Check sheet for the modelled part. Datum: model origin and axes. Units: mm. A direction names the side the tool comes from. Round coordinates to 2 decimals unless told otherwise and drop trailing zeros. Order: outer loops, then holes, each group sorted by start corner. A loop starts at its lowest first (then second) coordinate and runs counter-clockwise, first axis right, second up. Notation, with made-up numbers: (76.25, 88.25) -> (87.25, 88.25) arc R31 ccw to (87.25, 119.25) -> close; hole circle Ø10 at (75, -30.5). An arc over 180 degrees is marked (long way). Answer in a Markdown table with one row per item.
```python
from build123d import *

# Parameters (mm, degrees)
SKETCH_1_W          = 60
SKETCH_1_H          = 20
SKETCH_1_W_2        = 58
SKETCH_1_H_2        = 18
EXTRUDE_1_DEPTH     = 320
SKETCH_2_R          = 2
CUT_EXTRUDE_1_DEPTH = 327.190128606
SKETCH_4_R          = 1.5
CUT_EXTRUDE_2_DEPTH = 327.190128606
SKETCH_5_R          = 10
SKETCH_5_R_2        = 12.5
CUT_EXTRUDE_3_DEPTH = 327.190128606


with BuildPart() as part:
    # 草图1 → 拉伸-薄壁1 (new body)
    with BuildSketch(Plane.XY):
        with Locations((30, 10)):
            Rectangle(SKETCH_1_W, SKETCH_1_H)
        with Locations((30, 10)):
            Rectangle(SKETCH_1_W_2, SKETCH_1_H_2, mode=Mode.SUBTRACT)
    extrude(amount=EXTRUDE_1_DEPTH)

    # 草图2 → 切除-拉伸1 (cut, through all)
    with BuildSketch(Plane(origin=(0, 20, 0), x_dir=(1, 0, 0), z_dir=(0, 1, 0))):
        with Locations(Location((5, -145, 0), (0, 0, 270))):
            Circle(SKETCH_2_R)
        with Locations(Location((5, -175, 0), (0, 0, 270))):
            Circle(SKETCH_2_R)
        with Locations(Location((55, -175, 0), (0, 0, 90))):
            Circle(SKETCH_2_R)
        with Locations(Location((55, -145, 0), (0, 0, 90))):
            Circle(SKETCH_2_R)
        with Locations(Location((5, -115, 0), (0, 0, 270))):
            Circle(SKETCH_2_R)
        with Locations(Location((5, -205, 0), (0, 0, 90))):
            Circle(SKETCH_2_R)
        with Locations(Location((55, -205, 0), (0, 0, 270))):
            Circle(SKETCH_2_R)
        with Locations(Location((55, -115, 0), (0, 0, 90))):
            Circle(SKETCH_2_R)
        with Locations(Location((5, -5, 0), (0, 0, 270))):
            Circle(SKETCH_2_R)
        with Locations(Location((55, -5, 0), (0, 0, 270))):
            Circle(SKETCH_2_R)
        with Locations(Location((55, -25, 0), (0, 0, 270))):
            Circle(SKETCH_2_R)
        with Locations(Location((5, -25, 0), (0, 0, 270))):
            Circle(SKETCH_2_R)
        with Locations(Location((5, -295, 0), (0, 0, 90))):
            Circle(SKETCH_2_R)
        with Locations(Location((55, -295, 0), (0, 0, 90))):
            Circle(SKETCH_2_R)
        with Locations(Location((55, -315, 0), (0, 0, 90))):
            Circle(SKETCH_2_R)
        with Locations(Location((5, -315, 0), (0, 0, 90))):
            Circle(SKETCH_2_R)
    extrude(amount=-CUT_EXTRUDE_1_DEPTH, mode=Mode.SUBTRACT)

    # 草图4 → 切除-拉伸2 (cut, through all)
    with BuildSketch(Plane(origin=(60, 0, 0), x_dir=(0, 0, -1), z_dir=(1, 0, 0))):
        with Locations((-315, 10)):
            Circle(SKETCH_4_R)
        with Locations((-295, 10)):
            Circle(SKETCH_4_R)
        with Locations(Location((-25, 10, 0), (0, 0, 180))):
            Circle(SKETCH_4_R)
        with Locations(Location((-5, 10, 0), (0, 0, 180))):
            Circle(SKETCH_4_R)
    extrude(amount=-CUT_EXTRUDE_2_DEPTH, mode=Mode.SUBTRACT)

    # 草图5 → 切除-拉伸3 (cut, through all)
    with BuildSketch(Plane(origin=(0, 20, 0), x_dir=(1, 0, 0), z_dir=(0, 1, 0))):
        with Locations(Location((30, -160, 0), (0, 0, 270))):
            Circle(SKETCH_5_R)
        with Locations(Location((30, -130, 0), (0, 0, 270))):
            Circle(SKETCH_5_R_2)
        with Locations(Location((30, -190, 0), (0, 0, 90))):
            Circle(SKETCH_5_R_2)
        with Locations(Location((30, -75, 0), (0, 0, 270))):
            Circle(SKETCH_5_R_2)
        with Locations(Location((30, -15, 0), (0, 0, 270))):
            Circle(SKETCH_5_R)
        with Locations(Location((30, -305, 0), (0, 0, 90))):
            Circle(SKETCH_5_R)
        with Locations(Location((30, -245, 0), (0, 0, 90))):
            Circle(SKETCH_5_R_2)
    extrude(amount=-CUT_EXTRUDE_3_DEPTH, mode=Mode.SUBTRACT)


solid = part.part
```
(1) Tool access check on faces 1 (the flat face through (16, 20, 158)), 2 (the flat face through (42, 1, 158)). Record the directions out of +Z, -Z, +X, -X, +Y, -Y that give a thin tool (end or side, any length) a straight path to the whole face; none if there is none.
Solutions:
| item | result |
|---|---|
| face 1 | +Z, -Z, +X, -X, +Y |
| face 2 | +Z, -Z |
(2) Section check B-B on x = 13. Record the boundary of the cut face in (y, z).
Solutions:
| item | result |
|---|---|
| outline | (0, 0) -> (1, 0) -> (1, 320) -> (0, 320) -> close; (19, 0) -> (20, 0) -> (20, 320) -> (19, 320) -> close |
(3) Depth check by flat-ended pin: pin 1 Ø12 at (y, z) = (14, 132.5) entering from -X. Enter the tip coordinate at first touch or a pass-through.
Solutions:
| item | result |
|---|---|
| pin 1 | x = 0 |
(4) Scan lines: probe 1 along X at (y, z) = (0.7, 205); probe 2 along Y at (x, z) = (18.5, 49.5); probe 3 along X at (y, z) = (3.5, 193.5). Record each from-to range of solid material in increasing order. Write a range as from..to.
Solutions:
| item | result |
|---|---|
| probe 1 | 0..3, 7..53, 57..60 |
| probe 2 | 0..1, 19..20 |
| probe 3 | 0..1, 59..60 |
(5) Section check A-A on z = 190. Record the boundary of the cut face in (x, y).
Solutions:
| item | result |
|---|---|
| outline | (0, 0) -> (17.5, 0) -> (17.5, 1) -> (1, 1) -> (1, 19) -> (17.5, 19) -> (17.5, 20) -> (0, 20) -> close; (42.5, 0) -> (60, 0) -> (60, 20) -> (42.5, 20) -> (42.5, 19) -> (59, 19) -> (59, 1) -> (42.5, 1) -> close |
(6) Section check C-C on z = 238. Record the boundary of the cut face in (x, y), plus the area to 3 significant figures.
Solutions:
| item | result |
|---|---|
| outline | (0, 0) -> (19.64, 0) -> (19.64, 1) -> (1, 1) -> (1, 19) -> (19.64, 19) -> (19.64, 20) -> (0, 20) -> close; (40.36, 0) -> (60, 0) -> (60, 20) -> (40.36, 20) -> (40.36, 19) -> (59, 19) -> (59, 1) -> (40.36, 1) -> close |
| area | 115 mm^2 |
(7) Draft check along Z on faces 3 (the cylindrical face through (26.17, 0.507, 169.237)), 4 (the flat face through (21, 19.7, 320)), 5 (the flat face through (59, 10, 158)). Enter one of: pulls with the +Z half, pulls with the -Z half, needs draft (parallel to the pull), parting line crosses it, or undercut.
Solutions:
| item | result |
|---|---|
| face 3 | undercut |
| face 4 | pulls with the +Z half |
| face 5 | needs draft |
